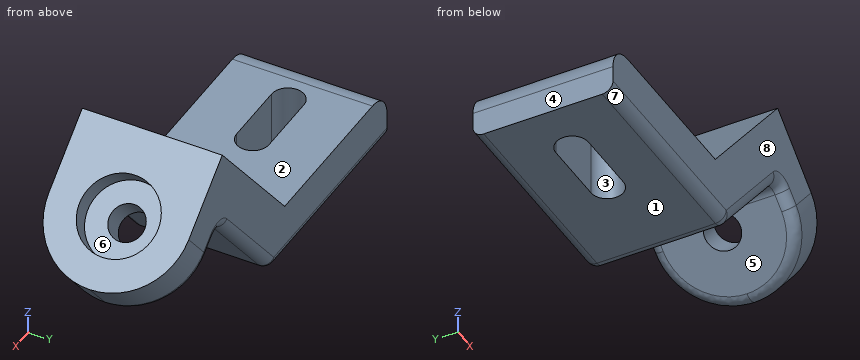
from build123d import *

# Parameters (mm, degrees)
F1_DEPTH    = 13
F2_T1_DEPTH = 75
F3_R        = 2
F4_R        = 7.3
F5_DEPTH    = 4.4
F6_R        = 3.3
F7_DEPTH    = 59.0732481421
F9_DEPTH    = 10.001
F10_R       = 5


# Not quite as in the source:
# - a fillet or chamfer that OpenCascade refuses, or shapes differently, is made with other operations: its cross-section is extruded or revolved along the edge and cut away or added


with BuildPart() as f1:
    # F0 (on Front) → F1 (new body, symmetric)
    with BuildSketch(Plane.XZ):
        Polygon((-38.8, 8), (-38.8, 0), (0, 0), (18.6408406809, 22.2152888505), (33.9617295433, 9.3595366567), (39.1040304208, 15.4878922017), (17.6547860135, 33.4859452729), (-3.7304612652, 8), align=None)
        Polygon((0, 0), (-38.8, 0), (-38.8, -2), (0.9326153163, -2), (18.8873543478, 19.3976247448), (32.6761543239, 7.8274477705), (33.9617295433, 9.3595366567), (18.6408406809, 22.2152888505), align=None)
    extrude(amount=F1_DEPTH, both=True)

    # F2: fillet of radius 13 on 2 edges, made by hand

    # F2_s2 → F2_t1 (cut)
    with BuildSketch(Plane(origin=(-3.5353318533, 0, -4.2132444372), x_dir=(0, 1, 0), z_dir=(0.6427876097, 0, 0.7660444431))):
        with BuildLine():
            ThreePointArc((0, -20), (-9.1923881554, -16.1923881554), (-13, -7))
            Line((-13, -7), (-13, -20))
            Line((-13, -20), (0, -20))
        make_face()
        with BuildLine():
            ThreePointArc((0, -20), (9.1923881554, -16.1923881554), (13, -7))
            Line((13, -7), (13, -20))
            Line((13, -20), (0, -20))
        make_face()
    extrude(amount=F2_T1_DEPTH, mode=Mode.SUBTRACT)

    # F3
    f3_edges = [f1.edges().sort_by_distance(p)[0] for p in [
        (18.887354, 0, 19.397625),
        (20.802465, -13, 17.790656),
        (29.759354, -9.192388, 10.274933),
        (29.759354, 9.192388, 10.274933),
        (20.802465, 13, 17.790656),
        (0.932615, 0, -2),
        (-18.933692, -13, -2),
        (-18.933692, 13, -2),
        (9.909985, 13, 8.698812),
        (9.909985, -13, 8.698812),
    ]]
    fillet(f3_edges, radius=F3_R)

    # F4 (on face) → F5 (cut)
    with BuildSketch(Plane(origin=(23.7831415584, 0, 28.3436443954), x_dir=(0.7660444431, 0, -0.6427876097), z_dir=(0.6427876097, 0, 0.7660444431))):
        with Locations((7, 0)):
            Circle(F4_R)
    extrude(amount=-F5_DEPTH, mode=Mode.SUBTRACT)

    # F6 (on face) → F7 (cut, through all)
    with BuildSketch(Plane(origin=(20.9548760758, 0, 24.9730488457), x_dir=(0.7660444431, 0, -0.6427876097), z_dir=(0.6427876097, 0, 0.7660444431))):
        with Locations((7, 0)):
            Circle(F6_R)
    extrude(amount=-F7_DEPTH, mode=Mode.SUBTRACT)

    # F8 (on face) → F9 (cut, through all)
    with BuildSketch(Plane.XY.offset(8)):
        with BuildLine():
            ThreePointArc((-28.8, 3), (-31.8, 0), (-28.8, -3))
            Line((-28.8, -3), (-16.8, -3))
            ThreePointArc((-16.8, -3), (-13.8, 0), (-16.8, 3))
            Line((-16.8, 3), (-28.8, 3))
        make_face()
    extrude(amount=-F9_DEPTH, mode=Mode.SUBTRACT)

    # F10
    f10_edges = [f1.edges().sort_by_distance(p)[0] for p in [
        (-38.8, 0, 8),
    ]]
    fillet(f10_edges, radius=F10_R)


solid = f1.part
Design review of the part built by this model. Coordinates are the model's own, in mm. Face numbers are marked on the shaded views. A direction names the side the tool comes from. Round coordinates to 2 decimals unless told otherwise and drop trailing zeros. Order: outer loops, then holes, each group sorted by start corner. A loop starts at its lowest first (then second) coordinate and runs counter-clockwise, first axis right, second up.
1) Clearance check with flat-ended pins moving along their axes: pin 1 Ø8 at (x, y) = (-24.5, -2) entering from +Z; pin 2 Ø6 at (x, z) = (28, 17) entering from -Y; pin 3 Ø12 at (x, z) = (-7.5, 11.5) entering from +Y; pin 4 Ø6 at (y, z) = (-9, 14) entering from -X. State where each tip first meets the part, or that it passes through.
The answers:
pin 1: stops at z = 8
pin 2: stops at y = -12.99
pin 3: stops at y = 13
pin 4: stops at x = -1.21
2) Consider section B-B (z = 17). Count the separate pieces of the cut face and the enclosed holes in it, plus the area to 3 significant figures.
The answers:
separate pieces: 2
enclosed holes: 1
area: 643 mm2
3) For L1, parallel to Y at x = -25.5, z = 0.5; L2, parallel to X at y = -3, z = 11.5; L3, parallel to X at y = 2.75, z = 6, list the stretches that pass through material, from the lowest coordinate up.
The answers:
L1: y = -13 to -3, 3 to 13
L2: x = -0.79 to 12.26, 28.3 to 35.3
L3: x = -37.8 to -30, -15.6 to 7.65
4) Consider section C-C (z = 29.5). State the section outline as (x, y) points, plus the area to 3 significant figures.
The answers:
outline: (14.31, -13) - (22.41, -13) - (22.41, 13) - (14.31, 13) - close
area: 210 mm2
5) Consider section A-A (x = -21.5). State the section outline as (y, z) points, plus the area to 3 significant figures.
The answers:
outline: (-13, 0) arc R2 ccw to (-11, -2) - (-3, -2) - (-3, 8) - (-13, 8) - close; (3, -2) - (11, -2) arc R2 ccw to (13, 0) - (13, 8) - (3, 8) - close
area: 198 mm2
6) Machinability: for the marked faces 1, 2, 3, 4 and 5, which of the approach directions +Z, -Z, +X, -X, +Y, -Y give a long, thin tool a straight path to every point of the face, cutting with its end or side? Answer none if there is none.
The answers:
face 1: -Z, +X, -X, +Y, -Y
face 2: +Z, -X, +Y, -Y
face 3: +Z, -Z
face 4: +Z, -Z, -X, +Y, -Y
face 5: -Z, +Y, -Y
7) Draft analysis for pull direction Z (two halves, no side actions). For the marked faces 6, 7 and 8, state which applies: released by +Z, released by -Z, zero draft, split by the parting line, or undercut.
The answers:
face 6: undercut
face 7: released by -Z
face 8: zero draft
